Work out the finished part from the listing and answer in its coordinate system (mm). A direction names the side the tool comes from. Give positions to 0.01 mm unless a question says otherwise; leave off trailing zeros. Order: outer loops, then holes, each group sorted by start corner. A loop starts at its lowest first (then second) coordinate and runs counter-clockwise, first axis right, second up. Notation, with made-up numbers: M 40,73 L 98,73 A30 ccw 98,112 Z; hole C -31,-16 d7. An arc over 180 degrees is marked long. One line per item, written item: value.
from build123d import *

# Parameters (mm, degrees)
F0_W     = 144.692793
F0_H     = 60.389988
F0_R     = 9.633917
F0_R_2   = 10.164922
F1_DEPTH = 25.4
F3_DEPTH = 61.214
F4_DEPTH = 6.35
F6_DEPTH = 8.128


with BuildPart() as f1:
    # F0 (on Top) → F1 (new body)
    with BuildSketch(Plane.XY):
        with Locations((0.991925, -9.922072)):
            Rectangle(F0_W, F0_H)
        with Locations((-52.305277, -10.124722)):
            Circle(F0_R, mode=Mode.SUBTRACT)
        with Locations((46.588395, -8.503514)):
            Circle(F0_R_2, mode=Mode.SUBTRACT)
    extrude(amount=F1_DEPTH)

    # F2 (on face) → F3 (cut)
    with BuildSketch(Plane.XZ.offset(40.117066)):
        with BuildLine():
            Line((23.738548, 25.4), (-17.442467, 25.4))
            ThreePointArc((-17.442467, 25.4), (3.148041, 20.508191), (23.738548, 25.4))
        make_face()
    extrude(amount=-F3_DEPTH, mode=Mode.SUBTRACT)

    # F2 (on face) → F4 (join)
    with BuildSketch(Plane.XZ.offset(40.117066)):
        with BuildLine():
            ThreePointArc((23.738548, 25.4), (3.148041, 20.508191), (-17.442467, 25.4))
            Line((-17.442467, 25.4), (-22.494383, 25.4))
            ThreePointArc((-22.494383, 25.4), (2.168844, 15.81733), (26.83207, 25.4))
            Line((26.83207, 25.4), (23.738548, 25.4))
        make_face()
    extrude(amount=F4_DEPTH)

    # F5 (on face) → F6 (join)
    with BuildSketch(Plane(origin=(0, 20.272922, 0), x_dir=(-1, 0, 0), z_dir=(0, 1, 0))):
        with BuildLine():
            Line((-23.738548, 25.4), (-26.600901, 25.4))
            ThreePointArc((-26.600901, 25.4), (-1.22531, 15.895824), (24.15028, 25.4))
            Line((24.15028, 25.4), (17.442467, 25.4))
            ThreePointArc((17.442467, 25.4), (-3.148041, 20.508191), (-23.738548, 25.4))
        make_face()
    extrude(amount=F6_DEPTH)


solid = f1.part
(1) Section D-D, the plane x = -19 is taken. Give the vertices of the cut face in (y, z).
Findings:
outline: M -46.47,22.58 L -40.12,22.58 L -40.12,0 L 20.27,0 L 20.27,21.61 L 28.4,21.61 L 28.4,25.4 L -46.47,25.4 Z
(2) Which of the six approach directions +Z, -Z, +X, -X, +Y, -Y give full straight-line access (tool end or side, diameter ignored) to faces 4 (the flat face through (0, 20.273, 13)), 5 (the cylindrical face through (1.79, -43.25, 15.82)), 6 (the flat face through (73.338, -10, 13))?
Findings:
face 4: -Z, +Y
face 5: -Z, -Y
face 6: +Z, -Z, +X, +Y, -Y
(3) Determine the mould class of faces 1 (the cylindrical face through (2.85, -9.56, 20.51)), 2 (the cylindrical face through (1.613, 24.28, 15.898)), 3 (the flat face through (54, -18, 25.4)) for opening direction X: pulls with the +X half, pulls with the -X half, needs draft (parallel to the pull), parting line crosses it, or undercut.
Findings:
face 1: undercut
face 2: parting line crosses it
face 3: needs draft
(4) Section B-B, the plane z = 3.25 is taken. Give the vertices of the cut face in (x, y), then the cut area to 3 significant figures.
Findings:
outline: M -71.35,-40.12 L 73.34,-40.12 L 73.34,20.27 L -71.35,20.27 Z; hole C -52.31,-10.12 d19.27; hole C 46.59,-8.5 d20.33
area: 8,120 mm^2
(5) Section A-A, the plane x = -47 is taken. Give the vertices of the cut face in (y, z).
Findings:
outline: M -40.12,0 L -18.17,0 L -18.17,25.4 L -40.12,25.4 Z; M -2.08,0 L 20.27,0 L 20.27,25.4 L -2.08,25.4 Z
(6) Given P1, Ø3, axis at x = -8.5, y = -0.5, coming from the +Z side; P2, Ø12, axis at x = -34, z = 18.5, coming from the +Y side; P3, Ø5, axis at x = -30, z = 9.5, coming from the -Y side; P4, Ø18.5, axis at x = 46.59, y = -8.5, coming from the +Z side, each flat-ended and moving along its own axis, determine where each tip first touches the part or whether it passes through.
Findings:
P1: stops at z = 22.44
P2: stops at y = 20.27
P3: stops at y = -40.12
P4: passes through
(7) Find the intervals of material crossed by probe 1 along X at (y, z) = (-15.5, 3.25); probe 2 along X at (y, z) = (-4.5, 7.75); probe 3 along Z at (x, y) = (20, -27), in increasing order. Write a range as from..to.
Findings:
probe 1: x = -71.35..-60.3, -44.31..39.21, 53.96..73.34
probe 2: x = -71.35..-60.13, -44.48..37.25, 55.93..73.34
probe 3: z = 0..23.72
(8) Section C-C, the plane y = -38.5 is taken. Give the vertices of the cut face in (x, z), then the cut area to 3 significant figures.
Findings:
outline: M -71.35,0 L 73.34,0 L 73.34,25.4 L 23.74,25.4 A45.78 cw -17.44,25.4 L -71.35,25.4 Z
area: 3,540 mm^2
